from build123d import *

# Parameters (mm, degrees)
SKETCH1_R           = 2.6
BOSS_EXTRUDE2_DEPTH = 5
BOSS_EXTRUDE3_DEPTH = 10
SKETCH1_5_W         = 5
SKETCH1_5_H         = 16
BOSS_EXTRUDE4_DEPTH = 25
FILLET1_R           = 8
FILLET2_R           = 8
FILLET3_R           = 8
FILLET4_R           = 8
FILLET5_R           = 8
FILLET6_R           = 8
SKETCH3_R           = 2.6
CUT_EXTRUDE1_DEPTH  = 25
SKETCH4_R           = 5
CUT_EXTRUDE2_DEPTH  = 1.5


# Some blends are built 0.0001 mm under size
with BuildPart() as part:
    # Sketch1 → Boss-Extrude2 (new body)
    with BuildSketch(Plane(origin=(0, 0, 0), x_dir=(1, 0, 0), z_dir=(0, 1, 0))):
        with BuildLine():
            Line((-25, 8), (-25, -8))
            Line((-25, -8), (14, -8))
            Line((14, -8), (14, -0.5))
            Line((14, -0.5), (10.06939799, -0.5))
            ThreePointArc((10.06939799, -0.5), (1.9, 0), (10.06939799, 0.5))
            Line((10.06939799, 0.5), (14, 0.5))
            Line((14, 0.5), (14, 8))
            Line((14, 8), (-25, 8))
        make_face()
        with Locations(Location((-15, 0, 0), (0, 0, 270))):
            Circle(SKETCH1_R, mode=Mode.SUBTRACT)
    extrude(amount=BOSS_EXTRUDE2_DEPTH)

    # Sketch1<4> → Boss-Extrude3 (add)
    with BuildSketch(Plane(origin=(0, 0, 0), x_dir=(1, 0, 0), z_dir=(0, 1, 0))):
        with BuildLine():
            Line((14, 8), (0, 8))
            Line((0, 8), (0, -8))
            Line((0, -8), (14, -8))
            Line((14, -8), (14, -0.5))
            Line((14, -0.5), (10.06939799, -0.5))
            ThreePointArc((10.06939799, -0.5), (1.9, 0), (10.06939799, 0.5))
            Line((10.06939799, 0.5), (14, 0.5))
            Line((14, 0.5), (14, 8))
        make_face()
    extrude(amount=BOSS_EXTRUDE3_DEPTH)

    # Sketch1<5> → Boss-Extrude4 (add)
    with BuildSketch(Plane(origin=(0, 0, 0), x_dir=(1, 0, 0), z_dir=(0, 1, 0))):
        with Locations((-2.5, 0)):
            Rectangle(SKETCH1_5_W, SKETCH1_5_H)
    extrude(amount=BOSS_EXTRUDE4_DEPTH)

    # Fillet1
    # the kernel refuses this fillet: 8 mm, written as the material it takes off along each edge
    with BuildSketch(Plane(origin=(14, 29.960899278, 8), x_dir=(0, 0, -1), z_dir=(0, -1, 0))) as fillet1_piece_1:
        with BuildLine():
            CenterArc((8, -7.984359711), FILLET1_R, 93.583321698, 86.416678302)
            Line((0, -7.984359711), (-0.16, -7.984359711))
            Line((-0.16, -7.984359711), (-0.16, 0))
            Line((-0.16, 0), (0, 0.16))
            ThreePointArc((0, 0.16), (3.75, 0.16), (7.49, 0.159687194))
            Line((7.49, 0.159687194), (7.5, 0))
        make_face()
    extrude(amount=49.921798557, mode=Mode.SUBTRACT)

    # Fillet2
    # the kernel refuses this fillet: 8 mm, written as the material it takes off along each edge
    with BuildSketch(Plane(origin=(14, -19.960899278, -8), x_dir=(0, 0, 1), z_dir=(0, 1, 0))) as fillet2_piece_1:
        with BuildLine():
            CenterArc((8, -7.984359711), FILLET2_R, 93.583321698, 86.416678302)
            Line((0, -7.984359711), (-0.16, -7.984359711))
            Line((-0.16, -7.984359711), (-0.16, 0))
            Line((-0.16, 0), (0, 0.16))
            ThreePointArc((0, 0.16), (3.75, 0.16), (7.49, 0.159687194))
            Line((7.49, 0.159687194), (7.5, 0))
        make_face()
    extrude(amount=49.921798557, mode=Mode.SUBTRACT)

    # Fillet3
    fillet3_edges = [part.edges().sort_by_distance(p)[0] for p in [
        (-25, 2.5, 8),
    ]]
    fillet(fillet3_edges, radius=FILLET3_R)

    # Fillet4
    fillet4_edges = [part.edges().sort_by_distance(p)[0] for p in [
        (-25, 2.5, -8),
    ]]
    fillet(fillet4_edges, radius=FILLET4_R - 0.0001)  # a hair under: the kernel refuses the full size

    # Fillet5
    fillet5_edges = [part.edges().sort_by_distance(p)[0] for p in [
        (-2.5, 25, 8),
    ]]
    fillet(fillet5_edges, radius=FILLET5_R)

    # Fillet6
    fillet6_edges = [part.edges().sort_by_distance(p)[0] for p in [
        (-2.5, 25, -8),
    ]]
    fillet(fillet6_edges, radius=FILLET6_R - 0.0001)  # a hair under: the kernel refuses the full size

    # Sketch3 → Cut-Extrude1 (cut)
    with BuildSketch(Plane.ZY.offset(5)):
        with Locations((0, 15)):
            Circle(SKETCH3_R)
    extrude(amount=-CUT_EXTRUDE1_DEPTH, mode=Mode.SUBTRACT)

    # Sketch4 → Cut-Extrude2 (cut)
    with BuildSketch(Plane(origin=(0, 0, 0), x_dir=(0, 0, -1), z_dir=(1, 0, 0))):
        with Locations((0, 15)):
            Circle(SKETCH4_R)
    extrude(amount=-CUT_EXTRUDE2_DEPTH, mode=Mode.SUBTRACT)


solid = part.part
For this review, take the finished solid that the model builds, in its own axes (mm). A direction names the side the tool comes from. Give positions to 0.01 mm unless a question says otherwise; leave off trailing zeros. Loops run counter-clockwise (first coordinate to the right, second up) from the corner with the lowest first, then second, coordinate; pieces in that order, holes last. Notation, with made-up numbers: (60.25, 47) - (93.25, 47) arc R34 ccw to (93.25, 84) - close; hole circle Ø3 at (-27, 26.25). An arc over 180 degrees is marked (long way). Write each question's results on one line, items separated by ' | '.
(1) Take a section at C-C (x = -14). Give the boundary of the cut face in (y, z), then the cut area to 3 significant figures.
Conclusion:
outline: (0, -8) - (5, -8) - (5, -2.4) - (0, -2.4) - close; (0, 2.4) - (5, 2.4) - (5, 8) - (0, 8) - close | area: 56.0 mm^2
(2) Draft analysis for pull direction Y (two halves, no side actions). For faces 1 (the flat face through (-1.5, 13, -2)), 2 (the flat face through (-3, 5, 8)), 3 (the flat face through (-13, 5, -2)), 4 (the cylindrical face through (-3.27, 12.46, -0.56)), state which applies: +Y half, -Y half, draft (parallel to the pull), parting line (faces both ways), or undercut.
Conclusion:
face 1: undercut | face 2: draft | face 3: +Y half | face 4: undercut
(3) For pin 1 Ø4 at (x, z) = (6.5, 5.5) entering from -Y; pin 2 Ø5 at (x, z) = (8, -0.5) entering from +Y; pin 3 Ø1.5 at (y, z) = (8, -5) entering from -X; pin 4 Ø3 at (x, z) = (-3.5, 4) entering from +Y, all flat-tipped, find the tip position at first contact; note any pin that passes through.
Conclusion:
pin 1: y = 0 | pin 2: y = 10 | pin 3: x = -5 | pin 4: y = 24.6
(4) For faces 5 (the flat face through (-5, 13, -2)), 6 (the cylindrical face through (-0.74, 10.12, 1.08)), 7 (the flat face through (0, 21, 0)), 8 (the flat face through (12, 5, -0.5)), list the 3-axis set-ups (+Z, -Z, +X, -X, +Y, -Y) from which the entire face can be reached by the end or side of a thin tool; tool diameter is ignored.
Conclusion:
face 5: +Z, -Z, -X, +Y | face 6: +X | face 7: +Z, -Z, +X, +Y | face 8: +X, +Y, -Y
(5) Take a section at D-D (y = 8.25). Give the boundary of the cut face in (x, z), then the cut area to 3 significant figures.
Conclusion:
outline: (-5, -8) - (6.02, -8) arc R8 ccw to (14, -0.5) - (10.07, -0.5) arc R4.1 cw (long way) to (10.07, 0.5) - (14, 0.5) arc R8 ccw to (6.02, 8) - (-5, 8) - close | area: 220 mm^2
(6) Take a section at B-B (z = -1.25). Give the boundary of the cut face in (x, y).
Conclusion:
outline: (-24.9, 0) - (-17.28, 0) - (-17.28, 5) - (-24.9, 5) - close; (-12.72, 0) - (2.1, 0) - (2.1, 10) - (0, 10) - (0, 10.16) - (-1.5, 10.16) - (-1.5, 12.72) - (-5, 12.72) - (-5, 5) - (-12.72, 5) - close; (-5, 17.28) - (-1.5, 17.28) - (-1.5, 19.84) - (0, 19.84) - (0, 24.9) - (-5, 24.9) - close; (9.9, 0) - (13.92, 0) - (13.92, 10) - (9.9, 10) - close
(7) For line 1 along Z through (x, y) = (-0.85, 15); line 2 along X through (y, z) = (11.5, 0.5); line 3 along X through (y, z) = (11, 7), list the stretches that pass through material, from the lowest coordinate up.
Conclusion:
line 1: -8 to -5, 5 to 8 | line 2: -5 to -1.5 | line 3: -5 to 0
